Source: CAD feature listing. Evaluate the final solid. Frame: model axes, mm. Face numbers are marked on the shaded views. A direction names the side the tool comes from. Give positions to 0.01 mm unless a question says otherwise; leave off trailing zeros. Loops run counter-clockwise (first coordinate to the right, second up) from the corner with the lowest first, then second, coordinate; pieces in that order, holes last. Notation, with made-up numbers: (88.25, 70) - (139.25, 70) arc R16 ccw to (139.25, 90) - close; hole circle Ø8 at (43.25, 89.25). An arc over 180 degrees is marked (long way). Write each question's results on one line, items separated by ' | '. Start each with the question number.
(1) Cut plane D-D on z = -31.5. Return the cut outline in (x, y).
(2) Pull-direction query (Z, two-part tool) for the marked faces 1, 2, 3 and 4; classes: pulls with the +Z half, pulls with the -Z half, needs draft (parallel to the pull), parting line crosses it, or undercut.
(3) Contact query for flat-ended pins moving along their axis: pin 1 (12 mm diameter, centred on y = -14, z = 11.5, fed in from +X); pin 2 (3.5 mm diameter, centred on y = -3.5, z = -33, fed in from -X); pin 3 (12 mm diameter, centred on x = -27, y = -9, fed in from -Z); pin 4 (8 mm diameter, centred on x = -21, z = -35.5, fed in from +Y). Output: stop coordinate, or through.
(4) Cut plane B-B on x = -6.5. Return the cut outline in (y, z).
(5) Material intervals for line 1 along Z through (x, y) = (0, -17.25); line 2 along X through (y, z) = (-9.5, 36); line 3 along Z through (x, y) = (0, -6), sorted ascending. Write a range as [from, to].
(6) Cut plane C-C on y = -17.25. Return the cut outline in (x, z).
(7) Reachability of the marked faces 5, 6, 7, 8 and 9 from +Z, -Z, +X, -X, +Y, -Y: full face, straight path, thin tool, end or side. Return the list, or none.
(8) Cut plane A-A on z = -12. Return the cut outline in (x, y), then the cut area to 3 significant figures.
from build123d import *

# Parameters (mm, degrees)
F0_R     = 47.222118
F0_R_2   = 26.321979
F0_R_3   = 14.082834
F1_DEPTH = 9.652
F2_R     = 24.729886
F2_R_2   = 14.082834
F3_DEPTH = 16.51
F5_DEPTH = 58.166


with BuildPart() as f1:
    # F0 (on Front) → F1 (new body)
    with BuildSketch(Plane.XZ):
        Circle(F0_R)
        Circle(F0_R_2, mode=Mode.SUBTRACT)
        Circle(F0_R_2)
        Circle(F0_R_3, mode=Mode.SUBTRACT)
    extrude(amount=F1_DEPTH)

    # F2 (on face) → F3 (join)
    with BuildSketch(Plane.XZ.offset(9.652)):
        Circle(F2_R)
        Circle(F2_R_2, mode=Mode.SUBTRACT)
    extrude(amount=F3_DEPTH)

    # F4 (on Front) → F5 (intersect)
    with BuildSketch(Plane.XZ):
        Polygon((7.006876, 42.021585), (0, 47.32769), (-4.933179, 41.77786), (-10.38732, 46.625983), (-13.874567, 39.002948), (-19.557085, 41.602482), (-22.87385, 34.352116), (-27.775111, 36.594255), (-27.775111, 28.21162), (-34.532256, 28.21162), (-34.532256, 20.81185), (-43.781966, 20.81185), (-38.23214, 11.562139), (-45.260107, 7.34536), (-40.852892, 0), (-45.260107, -10.020521), (-36.106034, -14.046655), (-40.616142, -24.30112), (-30.542885, -28.731529), (-30.542885, -38.3863), (-19.11607, -35.611387), (-16.889893, -44.778563), (-8.043921, -39.47098), (0, -46.711039), (6.51653, -39.47098), (13.908958, -46.124652), (19.732716, -34.99474), (30.832369, -39.47098), (30.832369, -28.731529), (38.848784, -28.731529), (38.848784, -18.961906), (44.244453, -15.724506), (40.163699, -8.923248), (46.964957, -4.842494), (44.059461, 0), (46.964957, 7.34536), (40.082078, 12.795433), (44.244453, 18.052081), (35.1489, 21.120174), (37.983977, 29.524937), (28.44544, 32.742457), (28.44544, 39.619595), (20.996165, 35.150031), (20.996165, 42.394508), (14.308761, 38.382066), (14.308761, 46.402715), align=None)
    extrude(amount=F5_DEPTH, mode=Mode.INTERSECT)


solid = f1.part
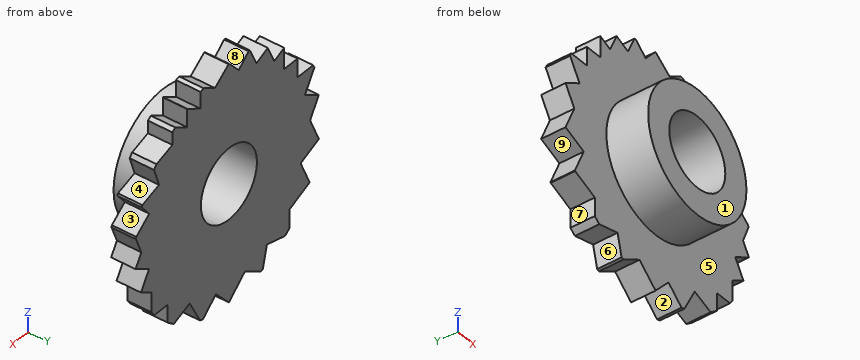
Ans:
1) outline: (-30.54, -9.65) - (30.83, -9.65) - (30.83, 0) - (-30.54, 0) - close
2) face 1: needs draft | face 2: pulls with the -Z half | face 3: undercut | face 4: undercut
3) pin 1: x = 46.64 | pin 2: x = -30.54 | pin 3: z = -37.83 | pin 4: y = 0
4) outline: (-26.16, -23.86) - (-9.65, -23.86) - (-9.65, -40.86) - (0, -40.86) - (0, -12.49) - (-26.16, -12.49) - close; (-26.16, 12.49) - (0, 12.49) - (0, 43.17) - (-9.65, 43.17) - (-9.65, 23.86) - (-26.16, 23.86) - close
5) line 1: [-24.73, -14.08], [14.08, 24.73] | line 2: [-27.78, -26.48], [-22.12, 21], [22.41, 28.45] | line 3: [-46.71, -14.08], [14.08, 47.22]
6) outline: circle Ø49.46 at (0, 0); hole circle Ø28.17 at (0, 0)
7) face 5: -Y | face 6: -Z, +Y, -Y | face 7: -Z, -X, +Y, -Y | face 8: +Z, +Y, -Y | face 9: -X, +Y, -Y
8) outline: (-40.76, -9.65) - (-21.62, -9.65) - (-21.62, -26.16) - (-7.37, -26.16) - (-7.37, 0) - (-40.76, 0) - close; (7.37, -26.16) - (21.62, -26.16) - (21.62, -9.65) - (42.01, -9.65) - (42.01, 0) - (7.37, 0) - close | area: 1,130 mm^2
